Drawing for the job (mm, zero at the part's lowest x, y, z). Give positions to 0.01 mm unless a question says otherwise; leave off trailing zeros. Order: outer loops, then holes, each group sorted by start corner. A loop starts at its lowest first (then second) coordinate and runs counter-clockwise, first axis right, second up. Notation, with made-up numbers: (0.5, 85.25) - (49.5, 85.25) arc R24 cw to (49.5, 118.25) - close; hole circle Ø4 at (45.5, -39.75). An arc over 180 degrees is marked (long way). Use CSV: the item, a comma, the result in double quotes. Start each with the question number.
(1) Band-saw the part on D-D, the plane x = 35. Give the cut face in (y, z).
(2) Band-saw the part on C-C, the plane z = 4.75. Give the cut face in (x, y), then the cut area to 3 significant figures.
(3) Probe L1, parallel to Y at x = 22.5, z = 2.5; L2, parallel to Y at x = 34, z = 0.5; L3, parallel to X at y = 3, z = 6.5. List the from-to ranges inside material, lowest first.
(4) Band-saw the part on B-B, the plane x = 10.5. Give the cut face in (y, z), then the cut area to 3 significant figures.
(5) Band-saw the part on A-A, the plane y = 50.5. Give the cut face in (x, z), then the cut area to 3 significant figures.
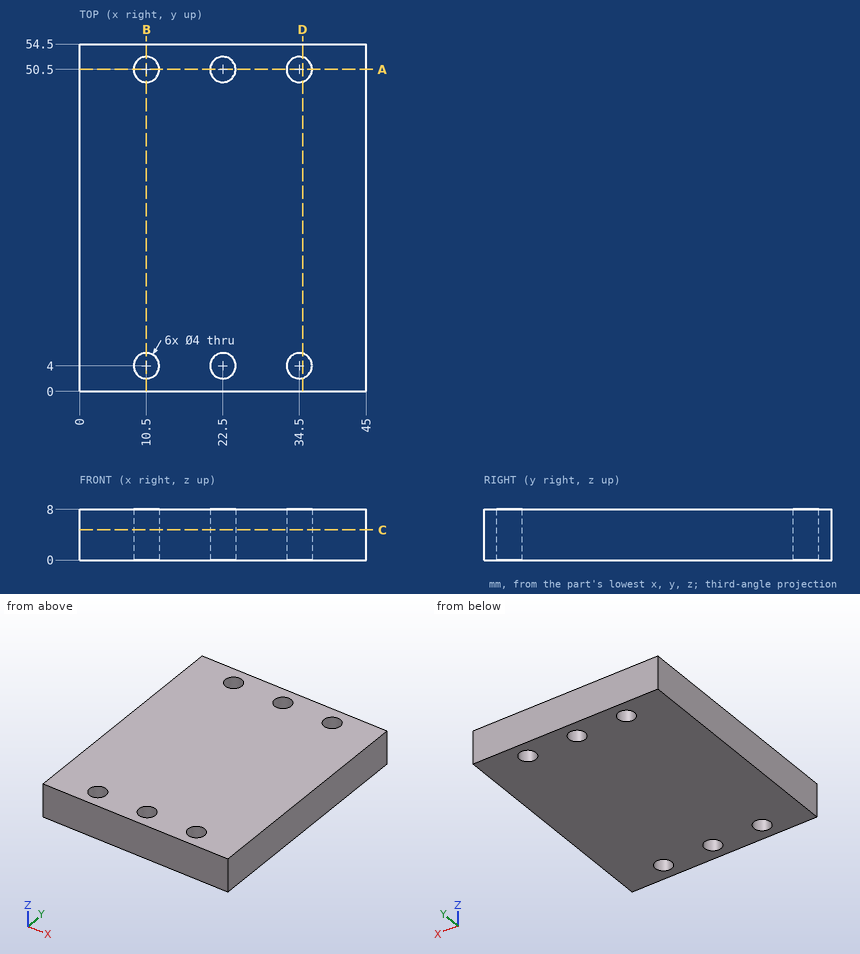
Answer block:
1,outline,"(0, 0) - (2.06, 0) - (2.06, 8) - (0, 8) - close; (5.94, 0) - (48.56, 0) - (48.56, 8) - (5.94, 8) - close; (52.44, 0) - (54.5, 0) - (54.5, 8) - (52.44, 8) - close"
2,outline,"(0, 0) - (45, 0) - (45, 54.5) - (0, 54.5) - close; hole circle Ø4 at (10.5, 4); hole circle Ø4 at (10.5, 50.5); hole circle Ø4 at (22.5, 4); hole circle Ø4 at (22.5, 50.5); hole circle Ø4 at (34.5, 4); hole circle Ø4 at (34.5, 50.5)"
2,area,"2,380 mm2"
3,L1,"y = 0 to 2, 6 to 48.5, 52.5 to 54.5"
3,L2,"y = 0 to 2.06, 5.94 to 48.56, 52.44 to 54.5"
3,L3,"x = 0 to 8.77, 12.23 to 20.77, 24.23 to 32.77, 36.23 to 45"
4,outline,"(0, 0) - (2, 0) - (2, 8) - (0, 8) - close; (6, 0) - (48.5, 0) - (48.5, 8) - (6, 8) - close; (52.5, 0) - (54.5, 0) - (54.5, 8) - (52.5, 8) - close"
4,area,"372 mm2"
5,outline,"(0, 0) - (8.5, 0) - (8.5, 8) - (0, 8) - close; (12.5, 0) - (20.5, 0) - (20.5, 8) - (12.5, 8) - close; (24.5, 0) - (32.5, 0) - (32.5, 8) - (24.5, 8) - close; (36.5, 0) - (45, 0) - (45, 8) - (36.5, 8) - close"
5,area,"264 mm2"
